Read the model definition and answer for the solid it produces. Units are mm, in the model's axes. A direction names the side the tool comes from. Give positions to 0.01 mm unless a question says otherwise; leave off trailing zeros. Loops run counter-clockwise (first coordinate to the right, second up) from the corner with the lowest first, then second, coordinate; pieces in that order, holes last. Notation, with made-up numbers: (79, 41.5) - (91, 41.5) arc R18 ccw to (91, 62.5) - close; hole circle Ø4 at (-35, 84). An arc over 180 degrees is marked (long way). Write item = value, one per line. Start each with the question number.
from build123d import *

# Parameters (mm, degrees)
F0_W     = 160
F0_H     = 150
F1_DEPTH = 20
F2_W     = 20
F2_H     = 150
F3_DEPTH = 10
F5_W     = 140
F5_H     = 4
F6_DEPTH = 3
F4_R     = 4
F7_DEPTH = 10


with BuildPart() as f1:
    # F0 (on Right) → F1 (new body)
    with BuildSketch(Plane.YZ):
        with Locations((-24.649234, 32.567439)):
            Rectangle(F0_W, F0_H)
    extrude(amount=F1_DEPTH)

    # F2 (on face) → F3 (cut)
    with BuildSketch(Plane(origin=(0, 0, 0), x_dir=(0, -1, 0), z_dir=(-1, 0, 0))):
        with Locations((-45.350766, 32.567439)):
            Rectangle(F2_W, F2_H)
    extrude(amount=-F3_DEPTH, mode=Mode.SUBTRACT)

    # F5 (on face) → F6 (cut)
    with BuildSketch(Plane(origin=(0, 0, 0), x_dir=(0, -1, 0), z_dir=(-1, 0, 0))):
        with Locations((34.649234, -34.432561)):
            Rectangle(F5_W, F5_H)
    extrude(amount=-F6_DEPTH, mode=Mode.SUBTRACT)

    # F4 (on face) → F7 (join)
    with BuildSketch(Plane.XZ.offset(104.649234)):
        with Locations((10, 72.067439)):
            Circle(F4_R)
        with Locations((10, 32.567439)):
            Circle(F4_R)
        with Locations((10, -6.932561)):
            Circle(F4_R)
    extrude(amount=F7_DEPTH)


solid = f1.part
1. A cutting plane is placed at A-A on z = 15.5. Give the vertices of the cut face in (x, y), and give its area (3 significant figures).
2. Given P1, Ø10, axis at x = 5.5, z = 57.5, coming from the -Y side; P2, Ø6, axis at y = 49, z = 34, coming from the -X side; P3, Ø10, axis at x = 2, z = -18, coming from the +Y side, each flat-ended and moving along its own axis, determine where each tip first touches the part or whether it passes through.
3. For a pull along Z with two mould halves and no side action, classify faces 5 (the flat face through (14.3, -104.649, 31.5)), 6 (the flat face through (0, -36, 39)), 7 (the flat face through (10, -26, -42.433)) as released by +Z, released by -Z, zero draft, split by the parting line, or undercut.
4. A cutting plane is placed at C-C on x = 17. Give the vertices of the cut face in (y, z), and give its area (3 significant figures).
5. Consider line 1 along Y through (x, z) = (5.5, 81); line 2 along Y through (x, z) = (15, -22); line 3 along X through (y, z) = (42, 55). Determine where each line is inside the solid, lowest interval first. Write a range as [from, to].
6. A cutting plane is placed at B-B on x = 8. Give the vertices of the cut face in (y, z).
7. A tool of negligible diameter and unlimited length cuts with its end or side. For faces 1 (the flat face through (5, 35.351, 32)), 2 (the flat face through (0, -36, -39)), 3 (the cylindrical face through (9.479, -109.579, 76.033)), 4 (the flat face through (3, -34, -34)), from which of +Z, -Z, +X, -X, +Y, -Y can it reach the whole face along a straight path? Write none if from no direction.
Reply:
q1.outline = (0, -104.65) - (20, -104.65) - (20, 55.35) - (10, 55.35) - (10, 35.35) - (0, 35.35) - close
q1.area = 3,000 mm^2
q2.P1 = -104.65
q2.P2 = 10
q2.P3 = 35.35
q3.face_5 = undercut
q3.face_6 = zero draft
q3.face_7 = released by -Z
q4.outline = (-104.65, -42.43) - (55.35, -42.43) - (55.35, 107.57) - (-104.65, 107.57) - close
q4.area = 24,000 mm^2
q5.line_1 = [-104.65, 35.35]
q5.line_2 = [-104.65, 55.35]
q5.line_3 = [10, 20]
q6.outline = (-114.65, -10.4) - (-104.65, -10.4) - (-104.65, -42.43) - (35.35, -42.43) - (35.35, 107.57) - (-104.65, 107.57) - (-104.65, 75.53) - (-114.65, 75.53) - (-114.65, 68.6) - (-104.65, 68.6) - (-104.65, 36.03) - (-114.65, 36.03) - (-114.65, 29.1) - (-104.65, 29.1) - (-104.65, -3.47) - (-114.65, -3.47) - close
q7.face_1 = +Z, -Z, -X, +Y
q7.face_2 = +Z, -Z, -X, +Y, -Y
q7.face_3 = -Y
q7.face_4 = -X, +Y, -Y
